```python
from build123d import *

# Parameters (mm, degrees)
SKETCH2_W             = 222.25
SKETCH2_H             = 254
BOSS_EXTRUDE1_DEPTH   = 3
SKETCH5_W             = 19.05
SKETCH5_H             = 3
SKETCH5_W_2           = 19.051189761
CUT_EXTRUDE1_DEPTH    = 4
F_4_CLEARANCE_HOLE2_D = 2.9464
SKETCH8_W             = 171.45
SKETCH8_H             = 139.7
CUT_EXTRUDE2_DEPTH    = 4


with BuildPart() as part:
    # Sketch2 → Boss-Extrude1 (new body)
    with BuildSketch(Plane(origin=(0, 0, 0), x_dir=(1, 0, 0), z_dir=(0, 1, 0))):
        with Locations((111.125, 127)):
            Rectangle(SKETCH2_W, SKETCH2_H)
    extrude(amount=BOSS_EXTRUDE1_DEPTH)

    # Sketch5 → Cut-Extrude1 (cut, through all)
    with BuildSketch(Plane(origin=(0, 3, 0), x_dir=(1, 0, 0), z_dir=(0, 1, 0))):
        with Locations((41.275, 249.5)):
            Rectangle(SKETCH5_W, SKETCH5_H)
        with Locations((73.025594881, 249.5)):
            Rectangle(SKETCH5_W_2, SKETCH5_H)
        with Locations((149.22440512, 249.5)):
            Rectangle(SKETCH5_W_2, SKETCH5_H)
        with Locations((180.975, 249.5)):
            Rectangle(SKETCH5_W, SKETCH5_H)
        with Locations((41.275, 4.5)):
            Rectangle(SKETCH5_W, SKETCH5_H)
        with Locations((73.025594881, 4.5)):
            Rectangle(SKETCH5_W_2, SKETCH5_H)
        with Locations((180.975, 4.5)):
            Rectangle(SKETCH5_W, SKETCH5_H)
        with Locations((149.22440512, 4.5)):
            Rectangle(SKETCH5_W_2, SKETCH5_H)
    extrude(amount=-CUT_EXTRUDE1_DEPTH, mode=Mode.SUBTRACT)

    # #4 Clearance Hole2 (through all)
    with Locations(Plane(origin=(0, 3, 0), x_dir=(1, 0, 0), z_dir=(0, 1, 0))):
        with Locations((57.15, 249.5), (165.1, 249.5), (165.1, 4.5), (57.15, 4.5)):
            Hole(F_4_CLEARANCE_HOLE2_D / 2)

    # Sketch8 → Cut-Extrude2 (cut, through all)
    with BuildSketch(Plane(origin=(0, 3, 0), x_dir=(1, 0, 0), z_dir=(0, 1, 0))):
        with Locations((111.125, 146.05)):
            Rectangle(SKETCH8_W, SKETCH8_H)
    extrude(amount=-CUT_EXTRUDE2_DEPTH, mode=Mode.SUBTRACT)


solid = part.part
```
Read the model definition and answer for the solid it produces. Units are mm, in the model's axes. Coordinates: 2 decimals unless noted, no trailing zeros. Loops run counter-clockwise (first coordinate to the right, second up) from the corner with the lowest first, then second, coordinate; pieces in that order, holes last.
(1) The part is cut by section C-C (y = 1.6). Count the separate pieces of the cut face and the enclosed holes in it, and give its area (3 significant figures).
Solution:
separate pieces: 1
enclosed holes: 13
area: 32,000 mm2
(2) Consider line 1 along Z through (x, y) = (57.15, 1.85); line 2 along Z through (x, y) = (28, 1.75); line 3 along X through (y, z) = (2.9, -138). Determine where each line is inside the solid, lowest interval first.
Solution:
line 1: z = -254 to -250.97, -248.03 to -215.9, -76.2 to -5.97, -3.03 to 0
line 2: z = -254 to -215.9, -76.2 to 0
line 3: x = 0 to 25.4, 196.85 to 222.25
(3) The part is cut by section A-A (z = -210). Determine the outline of the cut face in (x, y).
Solution:
outline: (0, 0) - (25.4, 0) - (25.4, 3) - (0, 3) - close; (196.85, 0) - (222.25, 0) - (222.25, 3) - (196.85, 3) - close
(4) The part is cut by section B-B (x = 178). Determine the outline of the cut face in (y, z), and give its area (3 significant figures).
Solution:
outline: (0, -254) - (3, -254) - (3, -251) - (0, -251) - close; (0, -248) - (3, -248) - (3, -215.9) - (0, -215.9) - close; (0, -76.2) - (3, -76.2) - (3, -6) - (0, -6) - close; (0, -3) - (3, -3) - (3, 0) - (0, 0) - close
area: 325 mm2
(5) A flat-ended cylindrical pin translates along its axis: pin 1 Ø2.5 at (x, z) = (165.1, -249.5) entering from -Y. Find the tip coordinate at first contact, or state that the pin passes through.
Solution:
pin 1: passes through
